from build123d import *

# Parameters (mm, degrees)
SKETCH1_W               = 96.89
SKETCH1_H               = 90.17
PCB_DEPTH               = 1.57
SKETCH2_R               = 2
M3_MOUNTING_HOLES_DEPTH = 1.57
SKETCH5_W               = 0.5
SKETCH5_H               = 90.17
CUT_EXTRUDE1_DEPTH      = 2.57
SKETCH6_W               = 3
SKETCH6_H               = 6
ZIPTIE_HOLDS_DEPTH      = 10


with BuildPart() as part:
    # Sketch1 → PCB (new body)
    with BuildSketch(Plane(origin=(0, 0, 0), x_dir=(1, 0, 0), z_dir=(0, 1, 0))):
        with Locations((16.200949951, 63.633996534)):
            Rectangle(SKETCH1_W, SKETCH1_H)
    extrude(amount=PCB_DEPTH)

    # Sketch2 → M3 Mounting Holes (cut)
    with BuildSketch(Plane(origin=(0, 1.57, 0), x_dir=(1, 0, 0), z_dir=(0, 1, 0))):
        with Locations((59.565949951, 24.898996534)):
            Circle(SKETCH2_R)
        with Locations((-26.164050049, 27.438996534)):
            Circle(SKETCH2_R)
        with Locations((-26.164050049, 101.098996534)):
            Circle(SKETCH2_R)
        with Locations((59.565949951, 103.638996534)):
            Circle(SKETCH2_R)
    extrude(amount=-M3_MOUNTING_HOLES_DEPTH, mode=Mode.SUBTRACT)

    # Sketch5 → Cut-Extrude1 (cut, through all)
    with BuildSketch(Plane(origin=(0, 1.57, 0), x_dir=(1, 0, 0), z_dir=(0, 1, 0))):
        with Locations((-31.994050049, 63.633996534)):
            Rectangle(SKETCH5_W, SKETCH5_H)
        with Locations((64.395949951, 63.633996534)):
            Rectangle(SKETCH5_W, SKETCH5_H)
    extrude(amount=-CUT_EXTRUDE1_DEPTH, mode=Mode.SUBTRACT)

    # Sketch6 → ZipTie Holds (cut)
    with BuildSketch(Plane(origin=(0, 1.57, 0), x_dir=(1, 0, 0), z_dir=(0, 1, 0))):
        with Locations((17.645949951, 85.718996534)):
            Rectangle(SKETCH6_W, SKETCH6_H)
        with Locations((47.645949951, 85.718996534)):
            Rectangle(SKETCH6_W, SKETCH6_H)
        with Locations((17.645949951, 45.718996534)):
            Rectangle(SKETCH6_W, SKETCH6_H)
        with Locations((47.645949951, 45.718996534)):
            Rectangle(SKETCH6_W, SKETCH6_H)
        with Locations((26.645949951, 27.548996534)):
            Rectangle(SKETCH6_W, SKETCH6_H)
        with Locations((38.645949951, 27.548996534)):
            Rectangle(SKETCH6_W, SKETCH6_H)
    extrude(amount=-ZIPTIE_HOLDS_DEPTH, mode=Mode.SUBTRACT)


solid = part.part
Part model, mm, in its own coordinate system. Give positions to 0.01 mm unless a question says otherwise; leave off trailing zeros. Loops run counter-clockwise (first coordinate to the right, second up) from the corner with the lowest first, then second, coordinate; pieces in that order, holes last. Notation, with made-up numbers: (33.5, 9.5) -> (43.5, 9.5) arc R28 ccw to (43.5, 45.5) -> close; hole circle Ø4 at (1, 34.5). An arc over 180 degrees is marked (long way). Write each question's results on one line, items separated by ' | '. Start each with the question number.
Q1. Wall check: L1, parallel to X at y = 0.3, z = -88; L2, parallel to X at y = 0.4, z = -29.5; L3, parallel to Z at x = 48.5, y = 1.45. Give the ranges that are in metal, low to high.
Q2. Band-saw the part on A-A on z = -85. List the corners of the cut face in (x, y).
Q3. Band-saw the part on B-B on y = 0.55. Count the separate pieces of the cut face and the enclosed holes in it, plus the area to 3 significant figures.
Q4. Pull direction Z, two halves, no side cores. Call faces 1 (the face through (60.489, 0.796, -101.865)), 2 (the face through (16, 1.57, -64)): +Z half, -Z half, draft (parallel to the pull), parting line (faces both ways), or undercut.
Results are:
1) L1: x = -31.74 to 16.15, 19.15 to 46.15, 49.15 to 64.15 | L2: x = -31.74 to 25.15, 28.15 to 37.15, 40.15 to 64.15 | L3: z = -108.72 to -88.72, -82.72 to -48.72, -42.72 to -18.55
2) outline: (-31.74, 0) -> (16.15, 0) -> (16.15, 1.57) -> (-31.74, 1.57) -> close; (19.15, 0) -> (46.15, 0) -> (46.15, 1.57) -> (19.15, 1.57) -> close; (49.15, 0) -> (64.15, 0) -> (64.15, 1.57) -> (49.15, 1.57) -> close
3) separate pieces: 1 | enclosed holes: 10 | area: 8,490 mm²
4) face 1: undercut | face 2: draft
